Verification items for the finished model (mm, model axes). Face numbers are marked on the shaded views. A direction names the side the tool comes from. Give positions to 0.01 mm unless a question says otherwise; leave off trailing zeros. Order: outer loops, then holes, each group sorted by start corner. A loop starts at its lowest first (then second) coordinate and runs counter-clockwise, first axis right, second up.
(1) Sectioned sample at D-D on x = -1.75. Record the cut outline in (y, z).
(2) Sectioned sample at C-C on z = 4. Record the cut outline in (x, y), plus the area to 3 significant figures.
(3) Gauge pin test, flat ends, axial feed: pin 1 (1.5 mm diameter, centred on x = -6.5, y = -11, fed in from +Z); pin 2 (5 mm diameter, centred on x = -9, y = -3, fed in from +Z); pin 3 (7 mm diameter, centred on y = 5, z = 9, fed in from -X). Record the tip position at first contact, or that the pin passes through.
(4) Scan lines: L1, parallel to X at y = -9.5, z = 17; L2, parallel to X at y = -8.35, z = 7.5 (3 decimals); L3, parallel to Z at x = 6, y = -8.3 (3 decimals). Record each from-to range of solid material in increasing order.
(5) Sectioned sample at B-B on x = -6. Record the cut outline in (y, z) (3 decimals), plus the area to 3 significant figures.
(6) Access from +Z, -Z, +X, -X, +Y, -Y to the whole of each face (thin tool, end or side, straight path). Record for the marked faces 1, 2 and 3.
(7) Sectioned sample at A-A on y = 6. Record the cut outline in (x, z) (3 decimals).
(8) Mould release check, pull along Z, two halves, no side actions. Record for the marked faces 4, 5, 6 and 7: pulls with the +Z half, pulls with the -Z half, needs draft (parallel to the pull), parting line crosses it, or undercut.
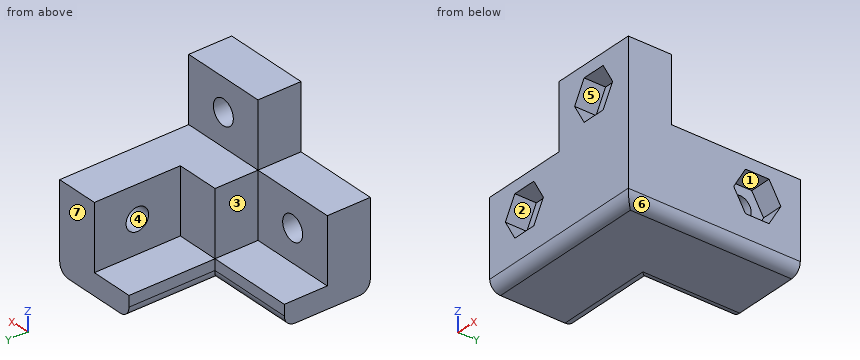
Autodesk Inventor part; units mm, degrees
ref_plane "YZ Plane" through (0, 0, 0) normal (1, 0, 0) x (0, 1, 0)
ref_plane "XZ Plane" through (0, 0, 0) normal (0, 1, 0) x (-1, 0, 0)
ref_plane "XY Plane" through (0, 0, 0) normal (0, 0, 1) x (1, 0, 0)
sketch "Sketch1" plane through (0, 0, 0) normal (0, 0, 1) x (1, 0, 0)
  line L0 (0, 0) -> (12, 0)
  line L1 (12, 0) -> (12, 12)
  line L2 (12, 12) -> (0, 12)
  line L3 (0, 12) -> (0, 0)
  line L4 (12, 0) -> (0, 0)
  line L5 (0, 0) -> (0, -12)
  line L6 (0, -12) -> (12, -12)
  line L7 (12, -12) -> (12, 0)
  line L8 (12, 0) -> (24, 0)
  line L9 (24, 0) -> (24, -12)
  line L10 (24, -12) -> (12, -12)
  line L11 (12, -12) -> (12, 0)
  line L12 (0, -12) -> (-12, -12)
  line L13 (-12, -12) -> (-12, 0)
  line L14 (-12, 0) -> (0, 0)
  line L15 (0, 0) -> (0, -12)
  line L16 (0, -12) -> (12, -12)
  line L17 (12, -12) -> (12, -24)
  line L18 (12, -24) -> (0, -24)
  line L19 (0, -24) -> (0, -12)
  dimension "d0" = 12
  dimension "d1" = 12
  dimension "d2" = 12
  dimension "d3" = 12
  dimension "d4" = 12
  dimension "d5" = 12
  dimension "d6" = 12
  dimension "d7" = 12
  dimension "d8" = 12
  dimension "d9" = 12
extrude "Extrusion1" add sketch "Sketch1" along normal blind 3
sketch "Sketch2" plane through (0, 0, 3) normal (0, 0, 1) x (1, 0, 0)
  line L0 (-12, 0) -> (-12, -12)
  line L1 (-12, -12) -> (-12, -6)
  line L2 (-12, -6) -> (0, -6)
  line L3 (-12, -12) -> (0, -12)
  line L4 (0, -6) -> (0, -12)
  line L5 (0, -12) -> (-12, -12)
  line L6 (12, -24) -> (12, -12)
  line L7 (12, -12) -> (12, -6)
  line L8 (12, -6) -> (24, -6)
  line L9 (24, -12) -> (24, 0)
  line L10 (12, -12) -> (24, -12)
  line L11 (24, -6) -> (24, -12)
  line L12 (24, -12) -> (12, -12)
  line L13 (0, 0) -> (0, -6)
  line L14 (12, 0) -> (12, 12)
  line L15 (0, 0) -> (12, 0)
  line L16 (12, 0) -> (12, -6)
  line L17 (12, -12) -> (0, -12)
  line L18 (0, 12) -> (0, 0)
  line L19 (0, 0) -> (0, 12)
  line L20 (0, 12) -> (6, 12)
  line L21 (12, 12) -> (0, 12)
  line L22 (6, 12) -> (6, 0)
  line L23 (6, 0) -> (0, 0)
  line L24 (0, -12) -> (0, -24)
  line L25 (0, -12) -> (0, -24)
  line L26 (0, -24) -> (6, -24)
  line L27 (0, -24) -> (12, -24)
  line L28 (6, -24) -> (6, -12)
  line L29 (6, -12) -> (0, -12)
  dimension "d12" = 6
  dimension "d13" = 12
extrude "Extrusion2" add sketch "Sketch2" along normal blind 9 contours L2 L4 L3 L0 | L13 L15 L16 L7 L17 L4 | L17 L28 L26 L24 | L18 L20 L22 L15 | L7 L8 L9 L10
sketch "Sketch3" plane through (0, 0, 12) normal (0, 0, 1) x (1, 0, 0)
  line L0 (0, -6) -> (12, -6)
  line L1 (12, -12) -> (6, -12)
  line L2 (12, -6) -> (12, -12)
  line L3 (0, -12) -> (0, -24)
  line L4 (12, -12) -> (0, -12)
  line L5 (0, -12) -> (0, -6)
  point P0 (0, 0)
extrude "Extrusion3" add sketch "Sketch3" along normal blind 9
sketch "Sketch4" plane through (6, -12, 3) normal (0, -1, 0) x (1, 0, 0)
  point P0 (-6, -3)
sketch "Sketch5" plane through (-12, -6, 3) normal (0, 1, 0) x (1, 0, 0)
  circle A0 centre (6, -4.5) radius 1.725
  line L0 (0, 0) -> (0, -9)
  line L1 (12, -9) -> (0, -9)
  circle A1 centre (18, -13.5) radius 1.725
  line L2 (24, -18) -> (12, -18)
  line L3 (24, -9) -> (24, -18)
  circle A2 centre (30, -4.5) radius 1.725
  line L4 (36, 0) -> (36, -9)
  line L5 (36, -9) -> (24, -9)
  point P0 (12, 3)
  dimension "d19" = 3.45
  dimension "d20" = 6
  dimension "d21" = 4.5
  dimension "d22" = 3.45
  dimension "d23" = 4.5
  dimension "d24" = 6
  dimension "d25" = 3.45
  dimension "d26" = 6
  dimension "d27" = 4.5
extrude "Extrusion4" cut sketch "Sketch5" against normal blind 3
sketch "Sketch6" plane through (6, -12, 3) normal (0, -1, 0) x (1, 0, 0)
  circle A0 centre (-12, 4.5) radius 1.725
  line L0 (-10.3546, 7.35) -> (-8.7091, 4.5)
  line L1 (-8.7091, 4.5) -> (-10.3546, 1.65)
  line L2 (-10.3546, 1.65) -> (-13.6454, 1.65)
  line L3 (-13.6454, 1.65) -> (-15.2909, 4.5)
  line L4 (-15.2909, 4.5) -> (-13.6454, 7.35)
  line L5 (-13.6454, 7.35) -> (-10.3546, 7.35)
  circle A1 centre (12, 4.5) radius 1.725
  line L6 (13.6454, 7.35) -> (15.2909, 4.5)
  line L7 (15.2909, 4.5) -> (13.6454, 1.65)
  line L8 (13.6454, 1.65) -> (10.3546, 1.65)
  line L9 (10.3546, 1.65) -> (8.7091, 4.5)
  line L10 (8.7091, 4.5) -> (10.3546, 7.35)
  line L11 (10.3546, 7.35) -> (13.6454, 7.35)
  circle A2 centre (0, 13.5) radius 1.725
  line L12 (1.6454, 16.35) -> (3.2909, 13.5)
  line L13 (3.2909, 13.5) -> (1.6454, 10.65)
  line L14 (1.6454, 10.65) -> (-1.6454, 10.65)
  line L15 (-1.6454, 10.65) -> (-3.2909, 13.5)
  line L16 (-3.2909, 13.5) -> (-1.6454, 16.35)
  line L17 (-1.6454, 16.35) -> (1.6454, 16.35)
  point P0 (-6, -3)
  dimension "d30" = 2.85
  dimension "d31" = 2.85
  dimension "d32" = 2.85
extrude "Extrusion5" cut sketch "Sketch6" against normal blind 3 contours A0 | L0 L1 L2 L3 L4 L5 | A1 | L6 L7 L8 L9 L10 L11 | A2 | L12 L13 L14 L15 L16 L17
sketch "Sketch7" plane through (6, 0, 3) normal (1, 0, 0) x (0, 0, -1)
  circle A0 centre (-4.5, 6) radius 1.725
  circle A1 centre (-4.5, -18) radius 1.725
  line L0 (-9, 0) -> (-9, 12)
  line L1 (-9, -24) -> (-9, -12)
  line L2 (0, -24) -> (-9, -24)
  line L3 (0, 12) -> (-9, 12)
  point P0 (3, 0)
  dimension "d35" = 3.45
  dimension "d36" = 3.45
  dimension "d37" = 4.5
  dimension "d38" = 4.5
  dimension "d39" = 6
  dimension "d40" = 6
extrude "Extrusion6" cut sketch "Sketch7" against normal blind 3
sketch "Sketch8" plane through (0, -6, 3) normal (-1, 0, 0) x (0, 0, 1)
  circle A0 centre (4.5, 12) radius 1.725
  line L0 (1.65, 13.6454) -> (4.5, 15.2909)
  line L1 (4.5, 15.2909) -> (7.35, 13.6454)
  line L2 (7.35, 13.6454) -> (7.35, 10.3546)
  line L3 (7.35, 10.3546) -> (4.5, 8.7091)
  line L4 (4.5, 8.7091) -> (1.65, 10.3546)
  line L5 (1.65, 10.3546) -> (1.65, 13.6454)
  circle A1 centre (4.5, -12) radius 1.725
  line L6 (1.65, -10.3546) -> (4.5, -8.7091)
  line L7 (4.5, -8.7091) -> (7.35, -10.3546)
  line L8 (7.35, -10.3546) -> (7.35, -13.6454)
  line L9 (7.35, -13.6454) -> (4.5, -15.2909)
  line L10 (4.5, -15.2909) -> (1.65, -13.6454)
  line L11 (1.65, -13.6454) -> (1.65, -10.3546)
  point P0 (-3, 6)
  dimension "d43" = 2.85
  dimension "d44" = 2.85
extrude "Extrusion7" cut sketch "Sketch8" against normal blind 3 contours A0 | L0 L1 L2 L3 L4 L5 | A1 | L6 L7 L8 L9 L10 L11
sketch "Sketch9" plane through (0, 0, 0) normal (0, 0, -1) x (-1, 0, 0)
  line L0 (-24, -12) -> (-24, 0)
  line L1 (-12, -12) -> (-12, -6)
  line L2 (-24, 0) -> (-12, 0)
  line L3 (-12, 0) -> (-12, -12)
  line L4 (-12, -12) -> (-24, -12)
  line L5 (-24, -12) -> (-24, 0)
  line L6 (-12, -12) -> (0, -12)
  line L7 (0, -12) -> (0, -24)
  line L8 (0, -24) -> (-12, -24)
  line L9 (-12, -24) -> (-12, -12)
  point P0 (0, 0)
extrude "Extrusion8" cut sketch "Sketch9" against normal through all
fillet "Fillet2" radius 1.5 4 edges at (12, 0, 0) (0, 6, 0) (-6, 0, 0) (0, -12, 0)
sketch "Sketch10" plane through (0, 12, 12) normal (0, 1, 0) x (1, 0, 0)
  line L0 (6, 0) -> (0, 0)
  line L1 (12, 9) -> (6, 9)
  line L2 (0, 0) -> (6, 0)
  line L3 (6, 0) -> (6, 9)
  line L4 (6, 9) -> (0, 9)
  line L5 (0, 9) -> (0, 0)
  point P0 (0, 12)
extrude "Extrusion9" cut sketch "Sketch10" against normal blind 12
sketch "Sketch11" plane through (0, 0, 3) normal (0, 1, 0) x (1, 0, 0)
  line L0 (12, 0) -> (12, -9)
  line L1 (12, 0) -> (0, 0)
  line L2 (12, -9) -> (6, -9)
  line L3 (6, -9) -> (6, 0)
  line L4 (6, 0) -> (12, 0)
  line L5 (12, 0) -> (12, -9)
  point P0 (0, 3)
extrude "Extrusion10" add sketch "Sketch11" along normal blind 12
sketch "Sketch12" plane through (6, 0, 3) normal (-1, 0, 0) x (0, 0, 1)
  circle A0 centre (4.5, 6) radius 1.575
  line L0 (9, 0) -> (9, 12)
  line L1 (0, 12) -> (9, 12)
  point P0 (-3, 0)
  dimension "d54" = 3.15
  dimension "d55" = 4.5
  dimension "d56" = 6
extrude "Extrusion11" cut sketch "Sketch12" against normal blind 3
sketch "Sketch13" plane through (12, -6, 12) normal (1, 0, 0) x (0, 0, -1)
  circle A0 centre (4.5, 12) radius 1.575
  line L0 (1.65, 13.6454) -> (4.5, 15.2909)
  line L1 (4.5, 15.2909) -> (7.35, 13.6454)
  line L2 (7.35, 13.6454) -> (7.35, 10.3546)
  line L3 (7.35, 10.3546) -> (4.5, 8.7091)
  line L4 (4.5, 8.7091) -> (1.65, 10.3546)
  line L5 (1.65, 10.3546) -> (1.65, 13.6454)
  point P0 (12, 6)
  dimension "d59" = 5.7
extrude "Extrusion12" cut sketch "Sketch13" against normal blind 3 contours A0 | L0 L1 L2 L3 L4 L5
properties part number "twoWayNEVer1"
Ans:
1. outline: (-12, 1.5) arc R1.5 ccw to (-10.5, 0) - (-1.5, 0) arc R1.5 ccw to (0, 1.5) - (0, 3) - (-6, 3) - (-6, 12) - (-12, 12) - close
2. outline: (-12, -12) - (12, -12) - (12, 12) - (6, 12) - (6, 0) - (0, 0) - (0, -6) - (-12, -6) - close
2. area: 288 mm2
3. pin 1: stops at z = 12
3. pin 2: stops at z = 3
3. pin 3: stops at x = 6
4. L1: x = 0 to 3, 9 to 12
4. L2: x = -12 to -7.725, -4.275 to 12
4. L3: z = 0 to 14.775, 18.225 to 21
5. outline: (-12, 1.5) arc R1.5 ccw to (-10.5, 0) - (-1.5, 0) arc R1.5 ccw to (0, 1.5) - (0, 3) - (-6, 3) - (-6, 5.775) - (-9, 5.775) - (-9, 4.65) - (-12, 4.65) - close; (-12, 10.35) - (-9, 10.35) - (-9, 9.225) - (-6, 9.225) - (-6, 12) - (-12, 12) - close
5. area: 61.6 mm2
6. face 1: +X
6. face 2: -Y
6. face 3: +Z, -X, +Y
7. outline: (0, 1.5) arc R1.5 ccw to (1.5, 0) - (10.5, 0) arc R1.5 ccw to (12, 1.5) - (12, 4.65) - (9, 4.65) - (9, 5.925) - (6, 5.925) - (6, 3) - (0, 3) - close; (6, 9.075) - (9, 9.075) - (9, 10.35) - (12, 10.35) - (12, 12) - (6, 12) - close
8. face 4: undercut
8. face 5: undercut
8. face 6: pulls with the -Z half
8. face 7: needs draft
